Could you check a few things on this model? Use its own coordinates, in mm. A direction names the side the tool comes from. Give positions to 0.01 mm unless a question says otherwise; leave off trailing zeros. Loops run counter-clockwise (first coordinate to the right, second up) from the corner with the lowest first, then second, coordinate; pieces in that order, holes last. Notation, with made-up numbers: (-10, 60.5) -> (0, 60.5) arc R18 ccw to (0, 86.5) -> close; hole circle Ø8 at (-33, 11). An arc over 180 degrees is marked (long way). Put each result on its own line as item: value.
Autodesk Fusion 360 part; units mm, degrees
sketch "Sketch1" plane through (0, 0, 0) normal (0, 0, 1) x (1, 0, 0)
  line L0 (27.32, 21.5) -> (-27.32, 21.5) construction
  line L1 (-27.32, 21.5) -> (-27.32, -21.5) construction
  line L2 (-27.32, -21.5) -> (27.32, -21.5) construction
  line L3 (27.32, -21.5) -> (27.32, 21.5) construction
  line L4 (27.32, 21.5) -> (-27.32, -21.5) construction
  line L5 (-27.32, 21.5) -> (27.32, -21.5) construction
  line L6 (-27.32, 21.246) -> (27.32, 21.246)
  line L7 (27.32, 21.246) -> (27.32, -21.246)
  line L8 (-27.32, 21.246) -> (-27.32, -21.246)
  line L9 (-27.32, 0) -> (0, 0) construction
  line L10 (-27.32, -21.246) -> (27.32, -21.246)
  dimension "d1" = 54.64
  dimension "d2" = 43
  dimension "d19" = 0.254
extrude "Extrude1" add sketch "Sketch1" along normal blind 2.513
sketch "Sketch2" plane through (0, 0, 0) normal (0, 0, -1) x (-1, 0, 0)
  line L0 (27.32, 21.246) -> (-4.355, 21.246)
  line L1 (-4.355, 21.246) -> (-4.355, -21.246)
  line L2 (-4.355, -21.246) -> (27.32, -21.246)
  line L3 (27.32, -21.246) -> (27.32, 21.246)
  line L4 (27.32, -21.246) -> (27.32, 21.246)
  line L5 (27.32, 21.246) -> (-27.32, 21.246)
  line L6 (-27.32, 21.246) -> (-27.32, -21.246)
  line L7 (-27.32, -21.246) -> (27.32, -21.246)
  dimension "d5" = 31.675
extrude "Extrude2" add sketch "Sketch2" along normal blind 2.987 contours L0 L1 L2 L3 L4 L5 L7
fillet "Fillet1" radius 3 2 edges at (27.32, 21.246, 1.2565) (27.32, -21.246, 1.2565)
sketch "Sketch5" plane through (0, 0, 0) normal (0, 0, -1) x (-1, 0, 0)
  line L0 (-4.355, 21.246) -> (-24.32, 21.246)
  arc A0 (-24.32, 21.246) -> (-27.32, 18.246) centre (-24.32, 18.246) ccw
  line L1 (-27.32, 18.246) -> (-27.32, -18.246)
  arc A1 (-27.32, -18.246) -> (-24.32, -21.246) centre (-24.32, -18.246) ccw
  line L2 (-24.32, -21.246) -> (-4.355, -21.246)
  line L3 (-20.54, 7) -> (-9.54, 7) construction
  line L4 (-9.54, 7) -> (-9.54, -7) construction
  line L5 (-9.54, -7) -> (-20.54, -7) construction
  line L6 (-20.54, -7) -> (-20.54, 7) construction
  line L7 (-27.32, 0) -> (-20.54, 0) construction
  line L8 (-9.794, -6.746) -> (-20.286, -6.746)
  line L9 (-20.286, -6.746) -> (-20.286, 6.746)
  line L10 (-20.286, 6.746) -> (-9.794, 6.746)
  line L11 (-9.794, 6.746) -> (-9.794, -6.746)
  line L12 (-4.355, -21.246) -> (-4.355, 21.246)
  dimension "d34" = 6.78
  dimension "d35" = 11
  dimension "d38" = 0.254
  dimension "d46" = 14
extrude "Extrude4" add sketch "Sketch5" along normal blind 2.9986 contours L8 L9 L10 L11
sketch "Sketch3" plane through (0, 0, 2.513) normal (0, 0, 1) x (1, 0, 0)
  line L0 (27.32, 21.5) -> (-27.32, 21.5) construction
  line L1 (-27.32, -21.5) -> (27.32, -21.5) construction
  line L2 (-27.32, 21.246) -> (-27.32, -21.246) construction
  line L3 (27.32, 21.246) -> (27.32, -21.246) construction
  line L4 (-27.32, 0) -> (0, 0) construction
  line L5 (0, 0) -> (27.32, 0) construction
  line L6 (15.04, 0) -> (15.04, 6.746) construction
  line L7 (9.794, 6.746) -> (20.286, 6.746) construction
  point P0 (-7.32, -15.5)
  point P1 (-7.32, 15.5)
  point P2 (15.04, 0)
  dimension "d25" = 6
  dimension "d28" = 20
hole "Hole1" at (-7.32, 15.5, 2.513) at (-7.32, -15.5, 2.513) at (15.04, 0, 2.513) direction (0, 0, -1) diameter 3.81 depth 39.751 tip angle 118 counterbore diameter 7.1374 counterbore depth 3.5052
fillet "Fillet2" radius 1.27 2 edges at (4.355, 0, 0) (4.355, 0, -2.987)
sketch "Sketch4" plane through (-27.32, 0, 0) normal (-1, 0, 0) x (0, 0, 1)
  line L0 (-2.987, -21.246) -> (2.513, -21.246)
  line L1 (2.513, -21.246) -> (2.513, 21.246)
  line L2 (2.513, 21.246) -> (-2.987, 21.246)
  line L3 (-2.987, 21.246) -> (-2.987, -21.246)
  line L4 (-2.3774, -4.0546) -> (-2.3774, 4.0546) construction
  line L5 (0, 0) -> (-2.3774, 0) construction
  line L6 (-2.987, 9.4361) -> (0.0102, 9.4361)
  line L7 (0.0102, 9.4361) -> (0.0102, -9.4361)
  line L8 (0.0102, -9.4361) -> (-2.987, -9.4361)
  line L9 (-2.987, -9.4361) -> (-2.987, 9.4361)
  line L10 (0, 0) -> (0.0102, 0) construction
  dimension "d30" = 2.3876
  dimension "d31" = 18.8722
  dimension "d41" = 0.6096
extrude "Extrude3" cut sketch "Sketch4" against normal blind 9.2964 contours L3 L6 L7 L8 L9
fillet "Fillet3" radius 1.5 4 edges at (20.286, 6.746, -1.4993) (9.794, 6.746, -1.4993) (20.286, -6.746, -1.4993) (9.794, -6.746, -1.4993)
sketch "Sketch6" plane through (0, 0, -2.987) normal (0, 0, -1) x (-1, 0, 0)
  circle A0 centre (7.32, 15.5) radius 1.905
  circle A1 centre (7.32, -15.5) radius 1.905
  line L0 (27.32, -9.4361) -> (18.0236, -9.4361)
  line L1 (18.0236, -9.4361) -> (18.0236, 9.4361)
  line L2 (18.0236, 9.4361) -> (27.32, 9.4361)
  line L3 (27.32, 9.4361) -> (27.32, 21.246)
  line L4 (27.32, 21.246) -> (-3.085, 21.246)
  line L5 (-3.085, 21.246) -> (-3.085, -21.246)
  line L6 (-3.085, -21.246) -> (27.32, -21.246)
  line L7 (27.32, -21.246) -> (27.32, -9.4361)
  line L8 (18.0236, 9.4361) -> (1.0236, 9.4361)
  line L9 (1.0236, 9.4361) -> (1.0236, -9.4361)
  line L10 (1.0236, -9.4361) -> (18.0236, -9.4361)
  line L11 (18.0236, -9.4361) -> (18.0236, 9.4361)
  line L12 (0, 0) -> (1.0236, 0) construction
  dimension "d43" = 17
extrude "Extrude5" cut sketch "Sketch6" against normal blind 2.2 contours L1 L8 L9 L10 L11
equation "d6 = 1.487 mm + 1.5 mm"
equation "d36 = 0.059 in + 1.5 mm"
1. I need wall thicknesses on line 1 (Y direction, x = -7.32, z = 1.3); line 2 (Y direction, x = -16, z = -1.05); line 3 (Y direction, x = -7.32, z = -1.4) (3 decimals). Which ranges of each line are inside material? Lowest first, please.
Recorded:
line 1: y = -21.25 to -19.07, -11.93 to 11.93, 19.07 to 21.25
line 2: y = -21.25 to -9.44, 9.44 to 21.25
line 3: y = -21.246 to -17.405, -13.595 to -9.436, 9.436 to 13.595, 17.405 to 21.246
2. If we section it at B-B (z = 1.2): List the corners of the cut face in (x, y) for me.
Recorded:
outline: (-27.32, -21.25) -> (24.32, -21.25) arc R3 ccw to (27.32, -18.25) -> (27.32, 18.25) arc R3 ccw to (24.32, 21.25) -> (-27.32, 21.25) -> close; hole circle Ø7.14 at (-7.32, -15.5); hole circle Ø7.14 at (-7.32, 15.5); hole circle Ø7.14 at (15.04, 0)
3. If we section it at C-C (y = 0): List the corners of the cut face in (x, z) for me (3 decimals), then the cut area to 3 significant figures.
Recorded:
outline: (-27.32, 0.01) -> (-18.024, 0.01) -> (-18.024, -0.787) -> (-1.024, -0.787) -> (-1.024, -2.987) -> (3.085, -2.987) arc R1.27 ccw to (4.355, -1.717) -> (4.355, -1.27) arc R1.27 cw to (5.625, 0) -> (9.794, 0) -> (9.794, -2.999) -> (13.135, -2.999) -> (13.135, -0.992) -> (11.471, -0.992) -> (11.471, 2.513) -> (-27.32, 2.513) -> close; (16.945, -2.999) -> (20.286, -2.999) -> (20.286, 0) -> (27.32, 0) -> (27.32, 2.513) -> (18.609, 2.513) -> (18.609, -0.992) -> (16.945, -0.992) -> close
area: 165 mm^2
4. If we section it at D-D (x = 15.04): List the corners of the cut face in (y, z) for me (3 decimals).
Recorded:
outline: (-21.246, 0) -> (-6.746, 0) -> (-6.746, -2.999) -> (-1.905, -2.999) -> (-1.905, -0.992) -> (-3.569, -0.992) -> (-3.569, 2.513) -> (-21.246, 2.513) -> close; (1.905, -2.999) -> (6.746, -2.999) -> (6.746, 0) -> (21.246, 0) -> (21.246, 2.513) -> (3.569, 2.513) -> (3.569, -0.992) -> (1.905, -0.992) -> close
5. If we section it at A-A (x = -7.32): List the corners of the cut face in (y, z) for me (3 decimals).
Recorded:
outline: (-21.246, -2.987) -> (-17.405, -2.987) -> (-17.405, -0.992) -> (-19.069, -0.992) -> (-19.069, 2.513) -> (-21.246, 2.513) -> close; (-13.595, -2.987) -> (-9.436, -2.987) -> (-9.436, -0.787) -> (9.436, -0.787) -> (9.436, -2.987) -> (13.595, -2.987) -> (13.595, -0.992) -> (11.931, -0.992) -> (11.931, 2.513) -> (-11.931, 2.513) -> (-11.931, -0.992) -> (-13.595, -0.992) -> close; (17.405, -2.987) -> (21.246, -2.987) -> (21.246, 2.513) -> (19.069, 2.513) -> (19.069, -0.992) -> (17.405, -0.992) -> close
6. Thinking about a two-plate mould opening in Y: for faces 5 (the face through (26.42, -20.39, 1.27)), 6 (the face through (-14, -9.436, -2)), 7 (the face through (0, 0, 2.513)), which applies, pulls with the +Y half, pulls with the -Y half, needs draft (parallel to the pull), parting line crosses it, or undercut?
Recorded:
face 5: pulls with the -Y half
face 6: undercut
face 7: needs draft
7. For faces 1 (the face through (15, 6.746, -1)), 2 (the face through (-5.8, 14, -0.992)), 3 (the face through (19.858, -6.295, -1.52)), 4 (the face through (-9, 0, -0.787)), which set-ups out of +Z, -Z, +X, -X, +Y, -Y let a thin tool reach every point of the face, with its end or its side?
Recorded:
face 1: -Z, +X, +Y
face 2: +Z
face 3: -Z, +X, -Y
face 4: -Z, -X
8. I'm going to push flat-ended pins straight in: pin 1 (8.5 mm diameter, centred on x = -5.5, y = 3.5, fed in from -Z); pin 2 (2 mm diameter, centred on x = 13, y = -11.5, fed in from -Z); pin 3 (5.5 mm diameter, centred on x = -7.32, y = 15.5, fed in from +Z). Where does each tip first touch, or does it pass through?
Recorded:
pin 1: stops at z = -0.79
pin 2: stops at z = 0
pin 3: stops at z = -0.99
